Verification items for the finished model (mm, model axes). Coordinates: 2 decimals unless noted, no trailing zeros. Write each loop counter-clockwise with the first axis right and the second up, starting at its lowest first coordinate (ties: lowest second). Pieces come first, ordered by that corner, then holes. Notation, with made-up numbers: (-29, 84.5) - (19, 84.5) arc R18 cw to (19, 90.5) - close; hole circle Ø1 at (-25, 25). An arc over 180 degrees is marked (long way). Answer as CSV lines item,"result". Start each with the question number.
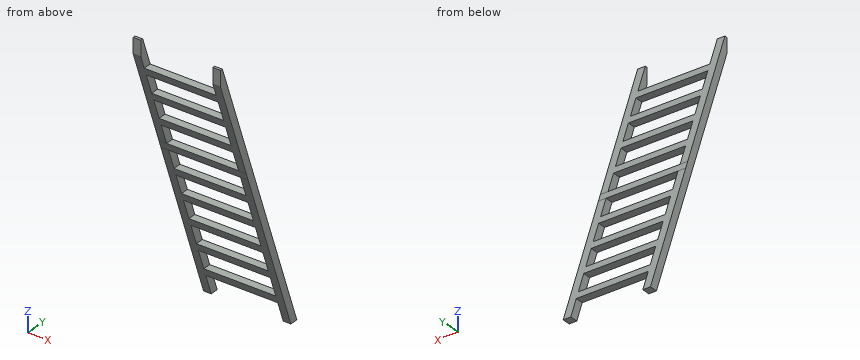
```python
from build123d import *

# Parameters (mm, degrees)
F1_DEPTH = 48
F3_DEPTH = 452


with BuildPart() as f1:
    # F0 (on Right) → F1 (new body)
    with BuildSketch(Plane.YZ):
        Polygon((538.1385763868, 312), (585.0655876551, 180), (636.0086209978, 180), (589.0816097296, 312), align=None)
        Polygon((457.0828296508, 540), (474.1471973847, 492), (525.0902307274, 492), (508.0258629935, 540), align=None)
        Polygon((265.1086926442, 1080), (282.1730603782, 1032), (333.1160937209, 1032), (316.051725987, 1080), align=None)
        Polygon((90.1989233716, 1572), (137.1259346399, 1440), (188.0689679826, 1440), (141.1419567144, 1572), align=None)
        Polygon((346.1644393803, 852), (393.0914506486, 720), (444.0344839913, 720), (397.1074727231, 852), align=None)
        Polygon((73.1345556377, 1620), (90.1989233716, 1572), (141.1419567144, 1572), (124.0775889805, 1620), align=None)
        Polygon((474.1471973847, 492), (521.0742086529, 360), (572.0172419957, 360), (525.0902307274, 492), align=None)
        Polygon((410.1558183825, 672), (457.0828296508, 540), (508.0258629935, 540), (461.0988517252, 672), align=None)
        Polygon((282.1730603782, 1032), (329.1000716464, 900), (380.0431049891, 900), (333.1160937209, 1032), align=None)
        Polygon((43.9829274256, 1702), (73.1345556377, 1620), (124.0775889805, 1620), (60.0862099783, 1800), (43.9829274256, 1800), align=None)
        Polygon((585.0655876551, 180), (602.129955389, 132), (653.0729887317, 132), (636.0086209978, 180), align=None)
        Polygon((393.0914506486, 720), (410.1558183825, 672), (461.0988517252, 672), (444.0344839913, 720), align=None)
        Polygon((602.129955389, 132), (649.0569666573, 0), (700, 0), (653.0729887317, 132), align=None)
        Polygon((201.1173136421, 1260), (218.181681376, 1212), (269.1247147187, 1212), (252.0603469848, 1260), align=None)
        Polygon((218.181681376, 1212), (265.1086926442, 1080), (316.051725987, 1080), (269.1247147187, 1212), align=None)
        Polygon((154.1903023738, 1392), (201.1173136421, 1260), (252.0603469848, 1260), (205.1333357165, 1392), align=None)
        Polygon((329.1000716464, 900), (346.1644393803, 852), (397.1074727231, 852), (380.0431049891, 900), align=None)
        Polygon((521.0742086529, 360), (538.1385763868, 312), (589.0816097296, 312), (572.0172419957, 360), align=None)
        Polygon((137.1259346399, 1440), (154.1903023738, 1392), (205.1333357165, 1392), (188.0689679826, 1440), align=None)
    extrude(amount=F1_DEPTH)


with BuildPart() as f2_1:
    # F2: copy of F1
    add(f1.part.moved(Location((-500, 0, 0))))


with BuildPart() as f1_1:
    add(f1.part)

    add(f2_1.part)  # F3 merges F2_1
    # F0 (on Right) → F3 (join)
    with BuildSketch(Plane.YZ):
        Polygon((585.0655876551, 180), (602.129955389, 132), (653.0729887317, 132), (636.0086209978, 180), align=None)
        Polygon((521.0742086529, 360), (538.1385763868, 312), (589.0816097296, 312), (572.0172419957, 360), align=None)
        Polygon((457.0828296508, 540), (474.1471973847, 492), (525.0902307274, 492), (508.0258629935, 540), align=None)
        Polygon((393.0914506486, 720), (410.1558183825, 672), (461.0988517252, 672), (444.0344839913, 720), align=None)
        Polygon((329.1000716464, 900), (346.1644393803, 852), (397.1074727231, 852), (380.0431049891, 900), align=None)
        Polygon((265.1086926442, 1080), (282.1730603782, 1032), (333.1160937209, 1032), (316.051725987, 1080), align=None)
        Polygon((201.1173136421, 1260), (218.181681376, 1212), (269.1247147187, 1212), (252.0603469848, 1260), align=None)
        Polygon((137.1259346399, 1440), (154.1903023738, 1392), (205.1333357165, 1392), (188.0689679826, 1440), align=None)
        Polygon((73.1345556377, 1620), (90.1989233716, 1572), (141.1419567144, 1572), (124.0775889805, 1620), align=None)
    extrude(amount=-F3_DEPTH)


solid = f1_1.part
```
1. Depth check by flat-ended pin: P1, Ø5, axis at x = -202, y = 464, coming from the +Z side; P2, Ø8, axis at x = -284.5, y = 483.5, coming from the -Z side; P3, Ø15.5, axis at x = -251.5, y = 430.5, coming from the +Z side. Enter the tip coordinate at first touch or a pass-through.
2. Cross-section at A-A (x = -272). Count the separate pieces of the cut face and the enclosed holes in it, and give its area (3 significant figures).
3. Scan lines: line 1 along Z through (x, y) = (-103.5, 221); line 2 along Z through (x, y) = (-369, 357); line 3 along Y through (x, z) = (16, 1515). Record each from-to range of solid material in increasing order. Write a range as from..to.
4. Cross-section at B-B (z = 768.5). Record the cut outline in (x, y).
5. Cross-section at C-C (y = 299). Record the cut outline in (x, z), and give its area (3 significant figures).
Completed:
1,P1,"stops at z = 540"
1,P2,"stops at z = 492"
1,P3,"stops at z = 720"
2,separate pieces,"9"
2,enclosed holes,"0"
2,area,"22,000 mm2"
3,line 1,"z = 1212..1260"
3,line 2,"z = 852..900"
3,line 3,"y = 110.46..161.41"
4,outline,"(-500, 375.85) - (-452, 375.85) - (-452, 426.79) - (-500, 426.79) - close; (0, 375.85) - (48, 375.85) - (48, 426.79) - (0, 426.79) - close"
5,outline,"(-500, 984.67) - (-452, 984.67) - (-452, 1032) - (0, 1032) - (0, 984.67) - (48, 984.67) - (48, 1127.96) - (0, 1127.96) - (0, 1080) - (-452, 1080) - (-452, 1127.96) - (-500, 1127.96) - close"
5,area,"35,500 mm2"
